from build123d import *

# Parameters (mm, degrees)
SKETCH1_W           = 100
SKETCH1_H           = 800
BOSS_EXTRUDE1_DEPTH = 40
FILLET1_RADIUS      = 50
FILLET1_LENGTH      = 40
FILLET2_RADIUS      = 50
FILLET2_LENGTH      = 40
CUT_EXTRUDE1_DEPTH  = 406.092582011
SKETCH3_W           = 15
SKETCH3_H           = 700
CUT_EXTRUDE2_DEPTH  = 10
SKETCH4_W           = 40
SKETCH4_H           = 40
BOSS_EXTRUDE2_DEPTH = 900
FILLET3_R           = 10


with BuildPart() as part:
    # Sketch1 → Boss-Extrude1 (new body)
    with BuildSketch(Plane.XY):
        Rectangle(SKETCH1_W, SKETCH1_H)
    extrude(amount=BOSS_EXTRUDE1_DEPTH)

    # Fillet1: full round fillet: the end face becomes a half cylinder, R = half its width
    fillet1_face = Plane((0, 400, 20), x_dir=(0, 0, 1), z_dir=(0, 1, 0))  # on the end face: x along it, z out of the body
    fillet1_slab = fillet1_face.offset(-FILLET1_RADIUS / 2) * Box(FILLET1_LENGTH, 2 * FILLET1_RADIUS, FILLET1_RADIUS, mode=Mode.PRIVATE)  # the body's end, R deep
    fillet1_round = Plane((0, 350, 20), x_dir=(0, 1, 0), z_dir=(0, 0, 1)) * Cylinder(FILLET1_RADIUS, FILLET1_LENGTH, mode=Mode.PRIVATE)  # its axis R under the face
    add(fillet1_slab - fillet1_round, mode=Mode.SUBTRACT)

    # Fillet2: full round fillet: the end face becomes a half cylinder, R = half its width
    fillet2_face = Plane((0, -400, 20), x_dir=(0, 0, 1), z_dir=(0, -1, 0))  # on the end face: x along it, z out of the body
    fillet2_slab = fillet2_face.offset(-FILLET2_RADIUS / 2) * Box(FILLET2_LENGTH, 2 * FILLET2_RADIUS, FILLET2_RADIUS, mode=Mode.PRIVATE)  # the body's end, R deep
    fillet2_round = Plane((0, -350, 20), x_dir=(0, -1, 0), z_dir=(0, 0, 1)) * Cylinder(FILLET2_RADIUS, FILLET2_LENGTH, mode=Mode.PRIVATE)  # its axis R under the face
    add(fillet2_slab - fillet2_round, mode=Mode.SUBTRACT)

    # Sketch2 → Cut-Extrude1 (cut, through all)
    with BuildSketch(Plane(origin=(0, 0, 0), x_dir=(-1, 0, 0), z_dir=(0, 0, -1))):
        with BuildLine():
            Line((-32.5, 350), (-32.5, -350))
            ThreePointArc((-32.5, -350), (0, -382.5), (32.5, -350))
            Line((32.5, -350), (32.5, 350))
            ThreePointArc((32.5, 350), (0, 382.5), (-32.5, 350))
        make_face()
    extrude(amount=-CUT_EXTRUDE1_DEPTH, mode=Mode.SUBTRACT)

    # Sketch3 → Cut-Extrude2 (cut)
    with BuildSketch(Plane(origin=(-32.5, 0, 0), x_dir=(0, 0, -1), z_dir=(1, 0, 0))):
        with Locations((-20, 0)):
            Rectangle(SKETCH3_W, SKETCH3_H)
    cut_extrude2 = extrude(amount=-CUT_EXTRUDE2_DEPTH, mode=Mode.SUBTRACT)

    # Mirror1: Cut-Extrude2 across plane
    add(cut_extrude2.mirror(Plane(origin=(0, 0, 0), x_dir=(0, 0, 1), z_dir=(1, 0, 0))), mode=Mode.SUBTRACT)

    # Sketch4 → Boss-Extrude2 (add)
    with BuildSketch(Plane(origin=(50, 0, 0), x_dir=(0, 0, -1), z_dir=(1, 0, 0))):
        with Locations((-20, 1.179779929)):
            Rectangle(SKETCH4_W, SKETCH4_H)
    extrude(amount=BOSS_EXTRUDE2_DEPTH)

    # Fillet3
    fillet3_edges = [part.edges().sort_by_distance(p)[0] for p in [
        (50, 21.179779929, 20),
        (50, -18.820220071, 20),
    ]]
    fillet(fillet3_edges, radius=FILLET3_R)


solid = part.part
Can you work these out from the model? Positions are in its coordinate system, mm. A direction names the side the tool comes from. Round coordinates to 2 decimals unless told otherwise and drop trailing zeros. Write each loop counter-clockwise with the first axis right and the second up, starting at its lowest first coordinate (ties: lowest second). Pieces come first, ordered by that corner, then holes. Notation, with made-up numbers: M 48,21.5 L 60,21.5 A18 cw 60,51.5 Z; hole C 8.25,4 d3. An arc over 180 degrees is marked long. Use CSV: the item, a comma, the result in double quotes.
(1) I need wall thicknesses on line 1 along X through (y, z) = (-168.5, 5); line 2 along X through (y, z) = (-137, 16.5); line 3 along Z through (x, y) = (37.5, -145). Which ranges of each line are inside material? Lowest first, please.
Check values:
line 1,"-50 to -32.5, 32.5 to 50"
line 2,"-50 to -42.5, 42.5 to 50"
line 3,"0 to 12.5, 27.5 to 40"
(2) Imagine slicing it at B-B (y = 201.5). Write out the boundary of the cut face in (x, z).
Check values:
outline,"M -50,0 L -32.5,0 L -32.5,12.5 L -42.5,12.5 L -42.5,27.5 L -32.5,27.5 L -32.5,40 L -50,40 Z; M 32.5,0 L 50,0 L 50,40 L 32.5,40 L 32.5,27.5 L 42.5,27.5 L 42.5,12.5 L 32.5,12.5 Z"
(3) Imagine slicing it at C-C (z = 6.5). Write out the boundary of the cut face in (x, y).
Check values:
outline,"M -50,-350 A50 ccw 50,-350 L 50,-28.82 A10 cw 60,-18.82 L 950,-18.82 L 950,21.18 L 60,21.18 A10 cw 50,31.18 L 50,350 A50 ccw -50,350 Z; hole M -32.5,-350 A32.5 ccw 32.5,-350 L 32.5,350 A32.5 ccw -32.5,350 Z"
(4) Imagine slicing it at A-A (x = 0). Write out the boundary of the cut face in (y, z), plus the area to 3 significant figures.
Check values:
outline,"M -400,0 L -382.5,0 L -382.5,40 L -400,40 Z; M 382.5,0 L 400,0 L 400,40 L 382.5,40 Z"
area,"1,400 mm^2"
(5) I'm going to push flat-ended pins straight in: pin 1 (3 mm diameter, centred on x = -38, z = 16.5, fed in from -Y); pin 2 (8 mm diameter, centred on x = 54.5, y = 189, fed in from +Z); pin 3 (10 mm diameter, centred on x = 524, z = 10, fed in from +Y); pin 4 (10 mm diameter, centred on y = 36.5, z = 6.5, fed in from +X). Where does each tip first touch, or does it pass through?
Check values:
pin 1,"y = -384.17"
pin 2,"through"
pin 3,"y = 21.18"
pin 4,"x = 50"
(6) Imagine slicing it at D-D (x = 646). Write out the boundary of the cut face in (y, z), plus the area to 3 significant figures.
Check values:
outline,"M -18.82,0 L 21.18,0 L 21.18,40 L -18.82,40 Z"
area,"1,600 mm^2"
(7) We'd pull the mould along Y, two halves only. Please class faces 4 (the flat face through (950, 1, 20)), 5 (the cylindrical face through (-0.715, 382.492, 19.72)), 6 (the flat face through (499, -18.82, 20)): +Y half, -Y half, draft (parallel to the pull), parting line (faces both ways), or undercut.
Check values:
face 4,"draft"
face 5,"undercut"
face 6,"-Y half"
(8) On a 3-axis mill with a long thin cutter (end or side, diameter ignored), from which of +Z, -Z, +X, -X, +Y, -Y can I reach the whole of each face in a straight line? I mean faces 1 (the flat face through (499, 21.18, 20)), 2 (the cylindrical face through (0.715, -382.492, 19.72)), 3 (the flat face through (50, -192, 20)). Say none if no direction works.
Check values:
face 1,"+Z, -Z, +X, +Y"
face 2,"+Z, -Z"
face 3,"+Z, -Z, +X, -Y"
